The model under review builds one solid part; all positions refer to its coordinate system, in mm. A direction names the side the tool comes from. Round coordinates to 2 decimals unless told otherwise and drop trailing zeros. Order: outer loops, then holes, each group sorted by start corner. A loop starts at its lowest first (then second) coordinate and runs counter-clockwise, first axis right, second up. Notation, with made-up numbers: M -19.75,1.5 L -7.75,1.5 A22 ccw -7.75,13.5 Z; hole C 82.25,19 d4. An arc over 180 degrees is marked long. One line per item, written item: value. Start each with the question number.
from build123d import *

# Parameters (mm, degrees)
SKETCH1_W                                    = 12
SKETCH1_H                                    = 12
SKETCH1_W_2                                  = 126
SKETCH1_H_2                                  = 140
BOSS_EXTRUDE2_DEPTH                          = 30
CBORE_FOR_M4_HEX_SOCKET_HEAD_CAP_SCR_2_COUNT = 2
CBORE_FOR_M4_HEX_SOCKET_HEAD_CAP_SCR_2_PITCH = 138
CBORE_FOR_M4_HEX_SOCKET_HEAD_CAP_SCR_3_COUNT = 2
CBORE_FOR_M4_HEX_SOCKET_HEAD_CAP_SCR_3_PITCH = 163.670400501
CBORE_FOR_M4_HEX_SOCKET_HEAD_CAP_SCR_4_COUNT = 2
CBORE_FOR_M4_HEX_SOCKET_HEAD_CAP_SCR_4_PITCH = 88
CHAMFER1_SIZE                                = 12
FILLET1_R                                    = 8
FILLET2_R                                    = 6
CUT_EXTRUDE2_DEPTH                           = 27
CUT_EXTRUDE3_DEPTH                           = 1
SKETCH11_W                                   = 80
SKETCH11_H                                   = 25
CUT_EXTRUDE4_DEPTH                           = 1.6
SKETCH12_W                                   = 80
SKETCH12_H                                   = 27
CUT_EXTRUDE5_DEPTH                           = 1.9
CUT_EXTRUDE6_DEPTH                           = 1.9
SKETCH14_R                                   = 6
CUT_EXTRUDE8_DEPTH                           = 2
CUT_EXTRUDE9_DEPTH                           = 3


# Some blends are built 0.0001 mm under size
with BuildPart() as part:
    # Sketch1 → Boss-Extrude2 (new body)
    with BuildSketch(Plane(origin=(0, 0, 0), x_dir=(1, 0, 0), z_dir=(0, 1, 0))):
        with Locations((-69, -44)):
            Rectangle(SKETCH1_W, SKETCH1_H)
        Rectangle(SKETCH1_W_2, SKETCH1_H_2)
        with Locations((-69, 44)):
            Rectangle(SKETCH1_W, SKETCH1_H)
        with Locations((69, 44)):
            Rectangle(SKETCH1_W, SKETCH1_H)
        with Locations((69, -44)):
            Rectangle(SKETCH1_W, SKETCH1_H)
    extrude(amount=BOSS_EXTRUDE2_DEPTH)

    # Sketch3 → CBORE for M4 Hex Socket Head Cap Screw1 (revolve, cut)
    with BuildSketch(Plane(origin=(-69, 30, 44), x_dir=(0, 0, 1), z_dir=(1, 0, 0))):
        Polygon((0, 0), (0, 30), (3, 30), (2.4, 29.4), (2.4, 14.4), (4, 14.4), (4, 0), align=None)
    cbore_for_m4_hex_socket_head_cap_screw1 = revolve(axis=Axis((-69, 36.35, 44), (0, -1, 0)), mode=Mode.SUBTRACT)

    # CBORE for M4 Hex Socket Head Cap Scr 2: CBORE for M4 Hex Socket Head Cap Screw1 ×2
    with Locations(*[(i * CBORE_FOR_M4_HEX_SOCKET_HEAD_CAP_SCR_2_PITCH, 0, 0) for i in range(1, CBORE_FOR_M4_HEX_SOCKET_HEAD_CAP_SCR_2_COUNT)]):
        add(cbore_for_m4_hex_socket_head_cap_screw1, mode=Mode.SUBTRACT)

    # CBORE for M4 Hex Socket Head Cap Scr 3: CBORE for M4 Hex Socket Head Cap Screw1 ×2
    with Locations(*[Vector(0.8431579538999365, 0, -0.537665941617351) * (i * CBORE_FOR_M4_HEX_SOCKET_HEAD_CAP_SCR_3_PITCH) for i in range(1, CBORE_FOR_M4_HEX_SOCKET_HEAD_CAP_SCR_3_COUNT)]):
        add(cbore_for_m4_hex_socket_head_cap_screw1, mode=Mode.SUBTRACT)

    # CBORE for M4 Hex Socket Head Cap Scr 4: CBORE for M4 Hex Socket Head Cap Screw1 ×2
    with Locations(*[(0, 0, -i * CBORE_FOR_M4_HEX_SOCKET_HEAD_CAP_SCR_4_PITCH) for i in range(1, CBORE_FOR_M4_HEX_SOCKET_HEAD_CAP_SCR_4_COUNT)]):
        add(cbore_for_m4_hex_socket_head_cap_screw1, mode=Mode.SUBTRACT)

    # Chamfer1
    # the kernel refuses this chamfer: 12 mm, written as the material it takes off along each edge
    with BuildSketch(Plane(origin=(-75, 30, 7.139804144), x_dir=(0.9996219169112969, 0.027495876610586497, 0), z_dir=(0, 0, 1)), Plane(origin=(-75, 30, -80.860195856), x_dir=(0.9996219169112969, 0.027495876610586497, 0), z_dir=(0, 0, 1)), Plane(origin=(75, 30, -7.139804144), x_dir=(-0.9996219169112969, 0.027495876610586497, 0), z_dir=(0, 0, -1)), Plane(origin=(75, 30, 80.860195856), x_dir=(-0.9996219169112969, 0.027495876610586497, 0), z_dir=(0, 0, -1))) as chamfer1_piece_1:
        Polygon((CHAMFER1_SIZE * 0.999621916911, -CHAMFER1_SIZE * 0.0274958766106), (-CHAMFER1_SIZE * 0.0274958766106, -CHAMFER1_SIZE * 0.999621916911), (0, 0), align=None)
    extrude(amount=73.720391711, mode=Mode.SUBTRACT)

    # Fillet1
    fillet1_edges = [part.edges().sort_by_distance(p)[0] for p in [
        (-63, 15, -70),
        (63, 15, -70),
        (63, 15, 70),
        (-63, 15, 70),
    ]]
    fillet(fillet1_edges, radius=FILLET1_R)

    # Fillet2
    fillet2_edges = [part.edges().sort_by_distance(p)[0] for p in [
        (-63, 15, 38),
        (-63, 15, -38),
        (-63, 15, -50),
        (63, 15, -50),
        (63, 15, -38),
        (63, 15, 38),
        (63, 15, 50),
        (-63, 15, 50),
        (-75, 9, 50),
        (-75, 9, 38),
        (-75, 9, -38),
        (-75, 9, -50),
        (75, 9, -50),
        (75, 9, -38),
        (75, 9, 38),
        (75, 9, 50),
    ]]
    fillet(fillet2_edges, radius=FILLET2_R - 0.0001)  # a hair under: the kernel refuses the full size

    # Sketch6 → Cut-Extrude2 (cut)
    with BuildSketch(Plane(origin=(0, 30, 0), x_dir=(1, 0, 0), z_dir=(0, 1, 0))):
        with BuildLine():
            Line((-58, 52), (-58, -52))
            ThreePointArc((-58, -52), (-57.121320344, -54.121320344), (-55, -55))
            Line((-55, -55), (-51, -55))
            ThreePointArc((-51, -55), (-48.878679656, -55.878679656), (-48, -58))
            Line((-48, -58), (-48, -62))
            ThreePointArc((-48, -62), (-47.121320344, -64.121320344), (-45, -65))
            Line((-45, -65), (45, -65))
            ThreePointArc((45, -65), (47.121320344, -64.121320344), (48, -62))
            Line((48, -62), (48, -58))
            ThreePointArc((48, -58), (48.878679656, -55.878679656), (51, -55))
            Line((51, -55), (55, -55))
            ThreePointArc((55, -55), (57.121320344, -54.121320344), (58, -52))
            Line((58, -52), (58, 52))
            ThreePointArc((58, 52), (57.121320344, 54.121320344), (55, 55))
            Line((55, 55), (51, 55))
            ThreePointArc((51, 55), (48.878679656, 55.878679656), (48, 58))
            Line((48, 58), (48, 62))
            ThreePointArc((48, 62), (47.121320344, 64.121320344), (45, 65))
            Line((45, 65), (-45, 65))
            ThreePointArc((-45, 65), (-47.121320344, 64.121320344), (-48, 62))
            Line((-48, 62), (-48, 58))
            ThreePointArc((-48, 58), (-48.878679656, 55.878679656), (-51, 55))
            Line((-51, 55), (-55, 55))
            ThreePointArc((-55, 55), (-57.121320344, 54.121320344), (-58, 52))
        make_face()
    extrude(amount=-CUT_EXTRUDE2_DEPTH, mode=Mode.SUBTRACT)

    # Sketch7 → Cut-Extrude3 (cut)
    with BuildSketch(Plane(origin=(0, 30, 0), x_dir=(1, 0, 0), z_dir=(0, 1, 0))):
        with BuildLine():
            Line((55, 68.4), (-55, 68.4))
            ThreePointArc((-55, 68.4), (-59.5254834, 66.5254834), (-61.4, 62))
            Line((-61.4, 62), (-61.4, 56))
            Line((-61.4, 56), (-61.4, 32))
            Line((-61.4, 32), (-61.4, -32))
            Line((-61.4, -32), (-61.4, -56))
            Line((-61.4, -56), (-61.4, -62))
            ThreePointArc((-61.4, -62), (-59.5254834, -66.5254834), (-55, -68.4))
            Line((-55, -68.4), (55, -68.4))
            ThreePointArc((55, -68.4), (59.5254834, -66.5254834), (61.4, -62))
            Line((61.4, -62), (61.4, -56))
            Line((61.4, -56), (61.4, -32))
            Line((61.4, -32), (61.4, 32))
            Line((61.4, 32), (61.4, 56))
            Line((61.4, 56), (61.4, 62))
            ThreePointArc((61.4, 62), (59.5254834, 66.5254834), (55, 68.4))
        make_face()
        with BuildLine():
            Line((55, 66.8), (-55, 66.8))
            ThreePointArc((-55, 66.8), (-58.39411255, 65.39411255), (-59.8, 62))
            Line((-59.8, 62), (-59.8, 56))
            Line((-59.8, 56), (-59.8, 32))
            Line((-59.8, 32), (-59.8, -32))
            Line((-59.8, -32), (-59.8, -56))
            Line((-59.8, -56), (-59.8, -62))
            ThreePointArc((-59.8, -62), (-58.39411255, -65.39411255), (-55, -66.8))
            Line((-55, -66.8), (55, -66.8))
            ThreePointArc((55, -66.8), (58.39411255, -65.39411255), (59.8, -62))
            Line((59.8, -62), (59.8, -56))
            Line((59.8, -56), (59.8, -32))
            Line((59.8, -32), (59.8, 32))
            Line((59.8, 32), (59.8, 56))
            Line((59.8, 56), (59.8, 62))
            ThreePointArc((59.8, 62), (58.39411255, 65.39411255), (55, 66.8))
        make_face(mode=Mode.SUBTRACT)
    extrude(amount=-CUT_EXTRUDE3_DEPTH, mode=Mode.SUBTRACT)

    # Sketch11 → Cut-Extrude4 (cut)
    with BuildSketch(Plane(origin=(0, 0, -70), x_dir=(-1, 0, 0), z_dir=(0, 0, -1))):
        with Locations((0, 17.5)):
            Rectangle(SKETCH11_W, SKETCH11_H)
    extrude(amount=-CUT_EXTRUDE4_DEPTH, mode=Mode.SUBTRACT)

    # Sketch12 → Cut-Extrude5 (cut)
    with BuildSketch(Plane.XY.offset(-65)):
        with Locations((0, 16.5)):
            Rectangle(SKETCH12_W, SKETCH12_H)
    extrude(amount=-CUT_EXTRUDE5_DEPTH, mode=Mode.SUBTRACT)

    # Sketch13 → Cut-Extrude6 (cut)
    with BuildSketch(Plane.XY.offset(-66.9)):
        with BuildLine():
            Line((-33, 29), (-2.5, 29))
            Line((-2.5, 29), (-2.5, 15.5))
            ThreePointArc((-2.5, 15.5), (-3.378679656, 13.378679656), (-5.5, 12.5))
            Line((-5.5, 12.5), (-30, 12.5))
            ThreePointArc((-30, 12.5), (-32.121320344, 13.378679656), (-33, 15.5))
            Line((-33, 15.5), (-33, 29))
        make_face()
        with BuildLine():
            Line((30, 12.5), (5.5, 12.5))
            ThreePointArc((5.5, 12.5), (3.378679656, 13.378679656), (2.5, 15.5))
            Line((2.5, 15.5), (2.5, 29))
            Line((2.5, 29), (33, 29))
            Line((33, 29), (33, 15.5))
            ThreePointArc((33, 15.5), (32.121320344, 13.378679656), (30, 12.5))
        make_face()
    extrude(amount=-CUT_EXTRUDE6_DEPTH, mode=Mode.SUBTRACT)

    # Sketch14 → Cut-Extrude8 (cut)
    with BuildSketch(Plane(origin=(0, 0, 65), x_dir=(-1, 0, 0), z_dir=(0, 0, -1))):
        with Locations((38, 15)):
            Circle(SKETCH14_R)
        with Locations((23, 15)):
            Circle(SKETCH14_R)
    extrude(amount=-CUT_EXTRUDE8_DEPTH, mode=Mode.SUBTRACT)

    # Sketch16 → Cut-Extrude9 (cut)
    with BuildSketch(Plane(origin=(0, 0, 67), x_dir=(-1, 0, 0), z_dir=(0, 0, -1))):
        with BuildLine():
            Line((40.5, 12.923344034), (40.5, 17.076655966))
            ThreePointArc((40.5, 17.076655966), (34.75, 15), (40.5, 12.923344034))
        make_face()
        with BuildLine():
            Line((25.5, 12.923344034), (25.5, 17.076655966))
            ThreePointArc((25.5, 17.076655966), (19.75, 15), (25.5, 12.923344034))
        make_face()
    extrude(amount=-CUT_EXTRUDE9_DEPTH, mode=Mode.SUBTRACT)


solid = part.part
Item 1: Machinability: for faces 4 (the cylindrical face through (64.804, 15.21, 36.289)), 5 (the cylindrical face through (-64.711, 15.21, -36.196)), 6 (the flat face through (58, 17, 1)), which of the approach directions +Z, -Z, +X, -X, +Y, -Y give a long, thin tool a straight path to every point of the face, cutting with its end or side? Answer none if there is none.
Item 2: The part is to be moulded in two halves that separate along Y. For faces 1 (the flat face through (-66, 27, 47)), 2 (the cylindrical face through (-19.75, 15.11, 68.48)), 3 (the cylindrical face through (-64.711, 15.21, 51.804)), say which applies: pulls with the +Y half, pulls with the -Y half, needs draft (parallel to the pull), parting line crosses it, or undercut.
Item 3: Consider section B-B, the plane z = 25. Give the boundary of the cut face in (x, y).
Item 4: Wall thickness on L1, parallel to Y at x = -23, z = 65.55; L2, parallel to X at y = 11.5, z = 44; L3, parallel to X at y = 10, z = -48.5: over which ranges is each line inside the solid? List them lowest first.
Item 5: Clearance check with flat-ended pins moving along their axes: P1, Ø1.5, axis at y = 21.5, z = 28, coming from the +X side; P2, Ø4, axis at y = 8.5, z = 48.5, coming from the +X side; P3, Ø10, axis at x = 10, y = 13.5, coming from the -Z side. State where each tip first meets the part, or that it passes through.
Item 6: Consider section A-A, the plane x = -23. Give the boundary of the cut face in (y, z).
Computed:
1. face 4: +X, +Y, -Y
1. face 5: -X, +Y, -Y
1. face 6: +Y
2. face 1: pulls with the +Y half
2. face 2: undercut
2. face 3: needs draft
3. outline: M -63,0 L 63,0 L 63,30 L 61.4,30 L 61.4,29 L 59.8,29 L 59.8,30 L 58,30 L 58,3 L -58,3 L -58,30 L -59.8,30 L -59.8,29 L -61.4,29 L -61.4,30 L -63,30 Z
4. L1: y = 0 to 9, 21 to 30
4. L2: x = -75 to -71.4, -66.6 to -58, 58 to 66.6, 71.4 to 75
4. L3: x = -72.97 to -58, 58 to 72.97
5. P1: stops at x = 63
5. P2: stops at x = 74.45
5. P3: stops at z = -68.4
6. outline: M 0,-70 L 5,-70 L 5,-68.4 L 12.5,-68.4 L 12.5,-66.9 L 3,-66.9 L 3,65 L 9,65 L 9,67 L 11.75,67 L 11.75,70 L 0,70 Z; M 18.25,67 L 21,67 L 21,65 L 30,65 L 30,66.8 L 29,66.8 L 29,68.4 L 30,68.4 L 30,70 L 18.25,70 Z
